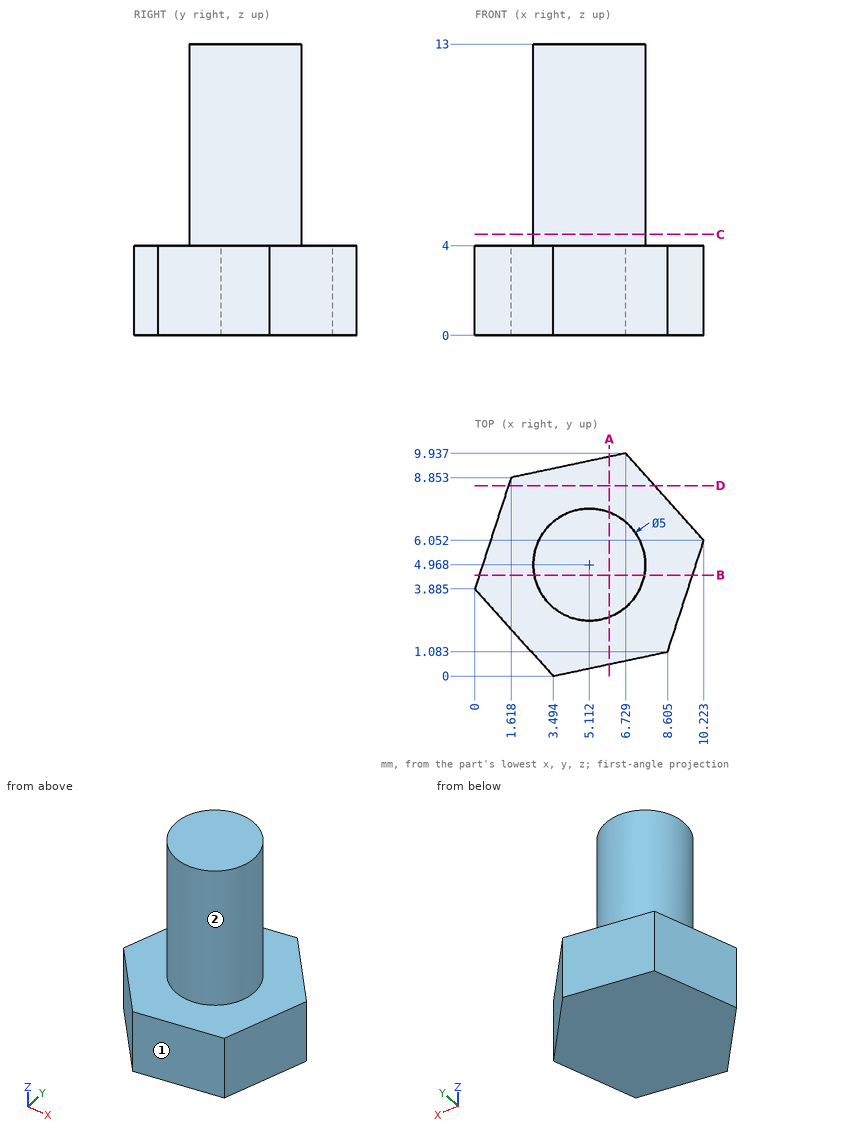
Answer from the drawing. Dimensions are ordinates in mm from the lowest x, y and z of the part. A direction names the side the tool comes from. Give positions to 0.01 mm unless a question says otherwise; leave off trailing zeros. Loops run counter-clockwise (first coordinate to the right, second up) from the corner with the lowest first, then second, coordinate; pieces in that order, holes last. Notation, with made-up numbers: (-18, 64.25) - (12, 64.25) arc R25 ccw to (12, 103.25) - close; hole circle Ø3 at (31.25, -11). An arc over 180 degrees is marked (long way). Write each question's results on one line, items separated by ' | '.
1. Flat-ended cylindrical pins translate along their axes: P1, Ø5, axis at y = 5, z = 10.5, coming from the -X side; P2, Ø3, axis at y = 8, z = 3, coming from the +X side; P3, Ø2, axis at x = 2.5, y = 1.5, coming from the +Z side. Find the tip coordinate at first contact, or state that the pin passes through.
Resolved:
P1: stops at x = 2.61 | P2: stops at x = 9.82 | P3: stops at z = 4
2. Find section C-C, the plane z = 4.5. Write down the section's boundary in (x, y).
Resolved:
outline: circle Ø5 at (5.11, 4.97)
3. Which of the six approach directions +Z, -Z, +X, -X, +Y, -Y give full straight-line access (tool end or side, diameter ignored) to the marked faces 1 and 2?
Resolved:
face 1: +Z, -Z, +X, -Y | face 2: +Z
4. Find section D-D, the plane y = 8.5. Write down the section's boundary in (x, z), then the cut area to 3 significant figures.
Resolved:
outline: (1.5, 0) - (8.02, 0) - (8.02, 4) - (1.5, 4) - close | area: 26.1 mm^2
5. Consider probe 1 along Z at (x, y) = (3.25, 7.25); probe 2 along Y at (x, z) = (5.25, 10) (1 decimal); probe 3 along Y at (x, z) = (2, 3.25) (1 decimal). Determine where each line is inside the solid, lowest interval first. Write a range as from..to.
Resolved:
probe 1: z = 0..4 | probe 2: y = 2.5..7.5 | probe 3: y = 1.7..8.9
6. Find section B-B, the plane y = 4.5. Write down the section's boundary in (x, z) (1 decimal).
Resolved:
outline: (0.2, 0) - (9.7, 0) - (9.7, 4) - (7.6, 4) - (7.6, 13) - (2.7, 13) - (2.7, 4) - (0.2, 4) - close
7. Find section A-A, the plane x = 6. Write down the section's boundary in (y, z) (1 decimal).
Resolved:
outline: (0.5, 0) - (9.8, 0) - (9.8, 4) - (7.3, 4) - (7.3, 13) - (2.6, 13) - (2.6, 4) - (0.5, 4) - close
